from build123d import *

# Parameters (mm, degrees)
F0_R     = 2
F1_DEPTH = 9.5
F0_R_2   = 4
F2_DEPTH = 8
F3_DEPTH = 2


with BuildPart() as f1:
    # F0 (on Top) → F1 (new body)
    with BuildSketch(Plane.XY):
        with BuildLine():
            Line((12.5, -20), (9.981460471, -8.3288922952))
            ThreePointArc((9.981460471, -8.3288922952), (0, -13), (-9.981460471, -8.3288922952))
            Line((-9.981460471, -8.3288922952), (-12.5, -20))
            Line((-12.5, -20), (0, -20))
            Line((0, -20), (12.5, -20))
        make_face()
        with Locations((-7.7868145891, -16.4918396622)):
            Circle(F0_R, mode=Mode.SUBTRACT)
        with Locations((7.7868145891, -16.4918396622)):
            Circle(F0_R, mode=Mode.SUBTRACT)
    extrude(amount=F1_DEPTH)



with BuildPart() as f2:
    # F0 (on Top) → F2 (new body)
    with BuildSketch(Plane.XY):
        Circle(F0_R_2)
    extrude(amount=F2_DEPTH)


with BuildPart() as f1_1:
    add(f1.part)

    add(f2.part)  # F3 merges F2
    # F0 (on Top) → F3 (join)
    with BuildSketch(Plane.XY):
        with BuildLine():
            Line((9.981460471, -8.3288922952), (7.8199968309, 1.6874980193))
            ThreePointArc((7.8199968309, 1.6874980193), (0, 8), (-7.8199968309, 1.6874980193))
            Line((-7.8199968309, 1.6874980193), (-9.981460471, -8.3288922952))
            ThreePointArc((-9.981460471, -8.3288922952), (0, -13), (9.981460471, -8.3288922952))
        make_face()
        Circle(F0_R_2, mode=Mode.SUBTRACT)
    extrude(amount=F3_DEPTH)


solid = f1_1.part
Build history of the part. All positions in model axes, mm. A direction names the side the tool comes from. Coordinates: 2 decimals unless noted, no trailing zeros. Order: outer loops, then holes, each group sorted by start corner. A loop starts at its lowest first (then second) coordinate and runs counter-clockwise, first axis right, second up. Notation, with made-up numbers: (53.5, -30) - (98.5, -30) arc R9 cw to (98.5, -17) - close; hole circle Ø4 at (86.5, 52). An arc over 180 degrees is marked (long way). Write item = value, one per line. Start each with the question number.
1) Saw through at B-B on x = 0. Write the cut outline in (y, z).
2) Saw through at A-A on z = 5. Write the cut outline in (x, y).
3) Saw through at D-D on y = 0. Write the cut outline in (x, z), then the cut area to 3 significant figures.
4) Saw through at C-C on x = 6.25. Write the cut outline in (y, z).
5) Flat gauge pins, fed straight in: pin 1 Ø4 at (y, z) = (-5.5, 5) entering from -X; pin 2 Ø2 at (x, y) = (6.5, -10) entering from +Z; pin 3 Ø1.5 at (y, z) = (-12.5, 7.5) entering from +X. Where does each tip first touch, or does it go through?
6) Wall check: line 1 along X through (y, z) = (-17.25, 5.5); line 2 along Z through (x, y) = (-3.25, 2); line 3 along Y through (x, z) = (2.5, 7.75). Give the ranges that are in metal, low to high. Write a range as from..to.
7) 3-axis set-ups, long thin cutter, end or side, ignore diameter. For faces 1 (the face through (0, 0, 8)), 2 (the face through (0, -5, 2)), 3 (the face through (0, 8, 1)): which of +Z, -Z, +X, -X, +Y, -Y reach the whole face in a straight line?
8) Two-plate mould, pull along Y, no slides. Class faces 4 (the face through (-9.26, -15.14, 4.68)), 5 (the face through (0, -20, 5)), 6 (the face through (0, -15, 9.5)), 7 (the face through (0, -13, 6)): pulls with the +Y half, pulls with the -Y half, needs draft (parallel to the pull), parting line crosses it, or undercut.
From the geometry:
q1.outline = (-20, 0) - (8, 0) - (8, 2) - (4, 2) - (4, 8) - (-4, 8) - (-4, 2) - (-13, 2) - (-13, 9.5) - (-20, 9.5) - close
q2.outline = (-12.5, -20) - (12.5, -20) - (9.98, -8.33) arc R13 cw to (-9.98, -8.33) - close; circle Ø8 at (0, 0); hole circle Ø4 at (-7.79, -16.49); hole circle Ø4 at (7.79, -16.49)
q3.outline = (-8.18, 0) - (8.18, 0) - (8.18, 2) - (4, 2) - (4, 8) - (-4, 8) - (-4, 2) - (-8.18, 2) - close
q3.area = 80.7 mm^2
q4.outline = (-20, 0) - (-17.77, 0) - (-17.77, 9.5) - (-20, 9.5) - close; (-15.21, 0) - (4.99, 0) - (4.99, 2) - (-11.4, 2) - (-11.4, 9.5) - (-15.21, 9.5) - close
q5.pin_1 = -1.94
q5.pin_2 = 2
q5.pin_3 = 11.04
q6.line_1 = -11.91..-9.64, -5.94..5.94, 9.64..11.91
q6.line_2 = 0..8
q6.line_3 = -20..-12.76, -3.12..3.12
q7.face_1 = +Z, +X, -X, +Y
q7.face_2 = +Z
q7.face_3 = +Z, -Z, +Y
q8.face_4 = undercut
q8.face_5 = pulls with the -Y half
q8.face_6 = needs draft
q8.face_7 = undercut
